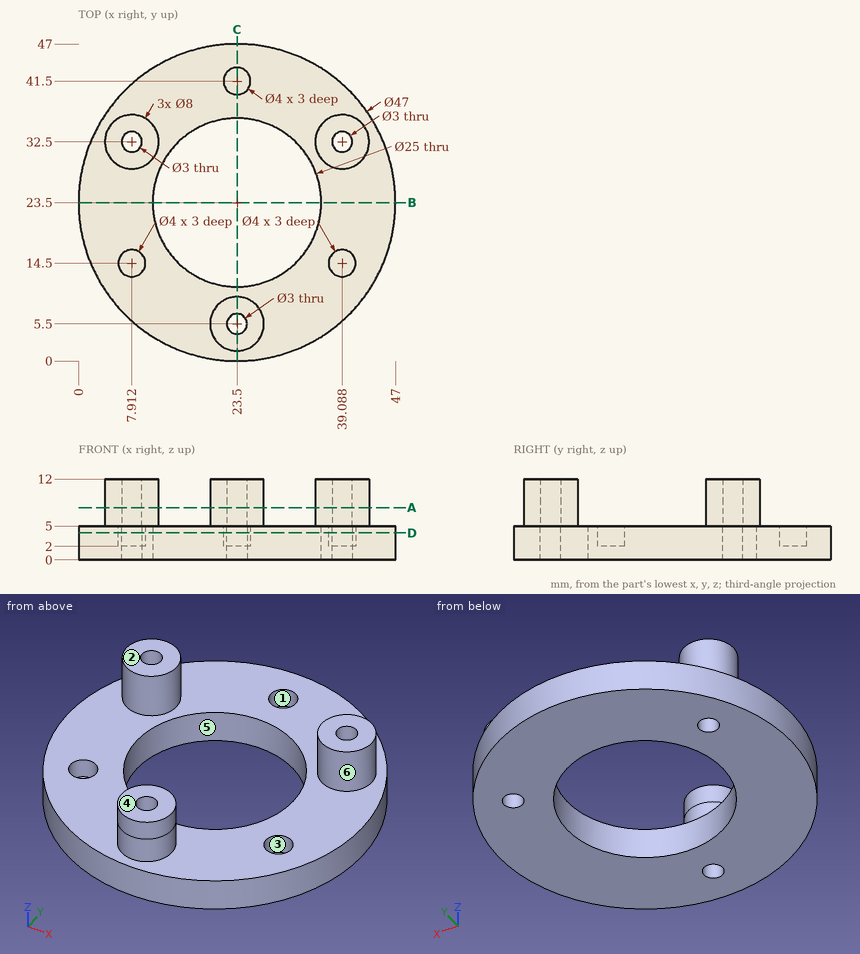
Verification items for this drawing (mm, ordinates from the low corner). A direction names the side the tool comes from. Give positions to 0.01 mm unless a question says otherwise; leave off trailing zeros. Loops run counter-clockwise (first coordinate to the right, second up) from the corner with the lowest first, then second, coordinate; pieces in that order, holes last.
1. Tool access check on the marked faces 1 and 2. Record the directions out of +Z, -Z, +X, -X, +Y, -Y that give a thin tool (end or side, any length) a straight path to the whole face; none if there is none.
Derived:
face 1: +Z
face 2: +Z, +X, -X, +Y, -Y
2. Cross-section at B-B on y = 23.5. Record the cut outline in (x, z).
Derived:
outline: (0, 0) - (11, 0) - (11, 5) - (0, 5) - close; (36, 0) - (47, 0) - (47, 5) - (36, 5) - close
3. Cross-section at D-D on z = 4. Record the cut outline in (x, y).
Derived:
outline: circle Ø47 at (23.5, 23.5); hole circle Ø4 at (7.91, 14.5); hole circle Ø3 at (7.91, 32.5); hole circle Ø25 at (23.5, 23.5); hole circle Ø4 at (23.5, 41.5); hole circle Ø3 at (23.5, 5.5); hole circle Ø4 at (39.09, 14.5); hole circle Ø3 at (39.09, 32.5)
4. Go/stop test with flat-tipped pins: P1, Ø4.5, axis at x = 22.5, y = 41, coming from the +Z side; P2, Ø3, axis at x = 11.5, z = 5, coming from the -Y side; P3, Ø2, axis at x = 40, y = 14.5, coming from the +Z side; P4, Ø22.5, axis at x = 23.5, y = 23.5, coming from the +Z side. Record where each tip stops, or that it passes through.
Derived:
P1: stops at z = 5
P2: stops at y = 2.48
P3: stops at z = 2
P4: passes through
5. Material ranges on probe 1 along Y at (x, z) = (23.5, 9.5); probe 2 along Y at (x, z) = (23.5, 3.85); probe 3 along Y at (x, z) = (13, 4) (1 decimal), recorded low to high.
Derived:
probe 1: y = 1.5 to 4, 7 to 9.5
probe 2: y = 0 to 4, 7 to 11, 36 to 39.5, 43.5 to 47
probe 3: y = 2.5 to 16.7, 30.3 to 44.5
6. Cross-section at A-A on z = 7.75. Record the cut outline in (x, y).
Derived:
outline: circle Ø8 at (7.91, 32.5); circle Ø8 at (23.5, 5.5); circle Ø8 at (39.09, 32.5); hole circle Ø3 at (7.91, 32.5); hole circle Ø3 at (23.5, 5.5); hole circle Ø3 at (39.09, 32.5)
7. Cross-section at C-C on x = 23.5. Record the cut outline in (y, z), and give its area (3 significant figures).
Derived:
outline: (0, 0) - (4, 0) - (4, 12) - (1.5, 12) - (1.5, 5) - (0, 5) - close; (7, 0) - (11, 0) - (11, 5) - (9.5, 5) - (9.5, 12) - (7, 12) - close; (36, 0) - (47, 0) - (47, 5) - (43.5, 5) - (43.5, 2) - (39.5, 2) - (39.5, 5) - (36, 5) - close
area: 118 mm2
8. Release check for a two-part mould opening along Y. For the marked faces 3, 4, 5 and 6 record: +Y half, -Y half, draft (parallel to the pull), parting line (faces both ways), or undercut.
Derived:
face 3: undercut
face 4: draft
face 5: undercut
face 6: parting line
